Could you check a few things on this model? Use its own coordinates, in mm. A direction names the side the tool comes from. Give positions to 0.01 mm unless a question says otherwise; leave off trailing zeros. Order: outer loops, then holes, each group sorted by start corner. A loop starts at its lowest first (then second) coordinate and runs counter-clockwise, first axis right, second up.
from build123d import *

# Parameters (mm, degrees)
BOSS_EXTRUDE1_DEPTH     = 88.9
SKETCH2_R               = 2.54
CUT_EXTRUDE1_DEPTH      = 4.445
F_1_4_CLEARANCE_HOLE1_D = 6.7564
BOSS_EXTRUDE3_DEPTH     = 6.35
SKETCH8_R               = 2.54
CUT_EXTRUDE2_DEPTH      = 4.445


with BuildPart() as part:
    # Sketch1 → Boss-Extrude1 (new body)
    with BuildSketch(Plane(origin=(0, 0, 0), x_dir=(1, 0, 0), z_dir=(0, 1, 0))):
        with BuildLine():
            Line((-17.78, 20.32), (7.62, 20.32))
            Line((7.62, 20.32), (7.62, 43.79198671))
            ThreePointArc((7.62, 43.79198671), (-8.864740287, 43.557076114), (-24.13, 37.33022368))
            Line((-24.13, 37.33022368), (-24.13, -37.33022368))
            ThreePointArc((-24.13, -37.33022368), (-8.864740287, -43.557076114), (7.62, -43.79198671))
            Line((7.62, -43.79198671), (7.62, -20.32))
            Line((7.62, -20.32), (-17.78, -20.32))
            Line((-17.78, -20.32), (-17.78, 20.32))
        make_face()
    extrude(amount=BOSS_EXTRUDE1_DEPTH)

    # Sketch2 → Cut-Extrude1 (cut)
    with BuildSketch(Plane(origin=(-17.78, 0, 0), x_dir=(0, 0, -1), z_dir=(1, 0, 0))):
        with Locations((-15.875, 76.2)):
            Circle(SKETCH2_R)
        with Locations((15.875, 76.2)):
            Circle(SKETCH2_R)
        with Locations((-15.875, 57.15)):
            Circle(SKETCH2_R)
        with Locations((15.875, 57.15)):
            Circle(SKETCH2_R)
        with Locations((-15.875, 38.1)):
            Circle(SKETCH2_R)
        with Locations((15.875, 38.1)):
            Circle(SKETCH2_R)
        with Locations((-15.875, 19.05)):
            Circle(SKETCH2_R)
        with Locations((15.875, 19.05)):
            Circle(SKETCH2_R)
    extrude(amount=-CUT_EXTRUDE1_DEPTH, mode=Mode.SUBTRACT)

    # 1/4 Clearance Hole1 (through all)
    with Locations(Plane(origin=(0, 88.9, 0), x_dir=(1, 0, 0), z_dir=(0, 1, 0))):
        with Locations((0, -25.4), (0, 25.4)):
            Hole(F_1_4_CLEARANCE_HOLE1_D / 2)

    # Sketch7 → Boss-Extrude3 (add)
    with BuildSketch(Plane.XZ):
        with BuildLine():
            Line((7.62, -20.32), (7.62, -43.79198671))
            ThreePointArc((7.62, -43.79198671), (44.45, 0), (7.62, 43.79198671))
            Line((7.62, 43.79198671), (7.62, 20.32))
            Line((7.62, 20.32), (-17.78, 20.32))
            Line((-17.78, 20.32), (-17.78, -20.32))
            Line((-17.78, -20.32), (7.62, -20.32))
        make_face()
    extrude(amount=-BOSS_EXTRUDE3_DEPTH)

    # Sketch8 → Cut-Extrude2 (cut)
    with BuildSketch(Plane(origin=(7.62, 0, 0), x_dir=(0, 0, -1), z_dir=(1, 0, 0))):
        with Locations((-34.925, 83.82)):
            Circle(SKETCH8_R)
        with Locations((34.925, 83.82)):
            Circle(SKETCH8_R)
        with Locations((-34.925, 11.43)):
            Circle(SKETCH8_R)
        with Locations((34.925, 11.43)):
            Circle(SKETCH8_R)
    extrude(amount=-CUT_EXTRUDE2_DEPTH, mode=Mode.SUBTRACT)


solid = part.part
Item 1: Imagine slicing it at B-B on y = 38.1. List the corners of the cut face in (x, z) for me (3 decimals).
Findings:
outline: (-24.13, -37.33) arc R44.45 ccw to (7.62, -43.792) - (7.62, -20.32) - (-17.78, -20.32) - (-17.78, -18.415) - (-22.225, -18.415) - (-22.225, -13.335) - (-17.78, -13.335) - (-17.78, 13.335) - (-22.225, 13.335) - (-22.225, 18.415) - (-17.78, 18.415) - (-17.78, 20.32) - (7.62, 20.32) - (7.62, 43.792) arc R44.45 ccw to (-24.13, 37.33) - close; hole circle Ø6.756 at (0, -25.4); hole circle Ø6.756 at (0, 25.4)
Item 2: Imagine slicing it at D-D on z = -25.4. List the corners of the cut face in (x, y) for me, then the cut area to 3 significant figures.
Findings:
outline: (-24.13, 0) - (-3.38, 0) - (-3.38, 88.9) - (-24.13, 88.9) - close; (3.38, 0) - (36.48, 0) - (36.48, 6.35) - (7.62, 6.35) - (7.62, 88.9) - (3.38, 88.9) - close
area: 2,410 mm2
Item 3: For pin 1 (4 mm diameter, centred on y = 58, z = 16.5, fed in from +X); pin 2 (4 mm diameter, centred on y = 38.1, z = -15.875, fed in from +X) (3 decimals); pin 3 (1.5 mm diameter, centred on y = 84.5, z = -34.5, fed in from +X) (3 decimals), each with a flat end and sliding along its axis, tell me the tip position at first contact or that it passes through.
Findings:
pin 1: stops at x = -17.78
pin 2: stops at x = -22.225
pin 3: stops at x = 3.175
Item 4: Imagine slicing it at A-A on x = 0. List the corners of the cut face in (y, z) for me, then the cut area to 3 significant figures.
Findings:
outline: (0, -44.45) - (88.9, -44.45) - (88.9, -28.78) - (0, -28.78) - close; (0, -22.02) - (88.9, -22.02) - (88.9, -20.32) - (6.35, -20.32) - (6.35, 20.32) - (88.9, 20.32) - (88.9, 22.02) - (0, 22.02) - close; (0, 28.78) - (88.9, 28.78) - (88.9, 44.45) - (0, 44.45) - close
area: 3,350 mm2
Item 5: Imagine slicing it at C-C on z = 15. List the corners of the cut face in (x, y) for me (3 decimals).
Findings:
outline: (-24.13, 0) - (41.843, 0) - (41.843, 6.35) - (-17.78, 6.35) - (-17.78, 16.665) - (-22.225, 16.665) - (-22.225, 21.435) - (-17.78, 21.435) - (-17.78, 35.715) - (-22.225, 35.715) - (-22.225, 40.485) - (-17.78, 40.485) - (-17.78, 54.765) - (-22.225, 54.765) - (-22.225, 59.535) - (-17.78, 59.535) - (-17.78, 73.815) - (-22.225, 73.815) - (-22.225, 78.585) - (-17.78, 78.585) - (-17.78, 88.9) - (-24.13, 88.9) - close
Item 6: For faces 3 (the flat face through (-17.78, 47, 0)), 4 (the cylindrical face through (5.429, 11.542, 37.463)), 5 (the flat face through (-19, 88.9, -1)), which set-ups out of +Z, -Z, +X, -X, +Y, -Y let a thin tool reach every point of the face, with its end or its side?
Findings:
face 3: +X, +Y
face 4: +X
face 5: +Z, -Z, +X, -X, +Y
Item 7: We'd pull the mould along Z, two halves only. Please class faces 1 (the cylindrical face through (-19.97, 54.67, -15.32)), 2 (the flat face through (-24.13, 44, -1)): +Z half, -Z half, draft (parallel to the pull), parting line (faces both ways), or undercut.
Findings:
face 1: undercut
face 2: draft
Item 8: Please list where these lines run through material, in increasing order: line 1 along Z through (x, y) = (-18, 19); line 2 along X through (y, z) = (46, 10); line 3 along Y through (x, z) = (27, 3.5).
Findings:
line 1: z = -40.64 to -18.41, -13.34 to 13.34, 18.41 to 40.64
line 2: x = -24.13 to -17.78
line 3: y = 0 to 6.35
